Geometry check sheet. Reference: drawing and pictorial views, mm from the part's lowest x, y, z. Give positions to 0.01 mm unless a question says otherwise; leave off trailing zeros. Loops run counter-clockwise (first coordinate to the right, second up) from the corner with the lowest first, then second, coordinate; pieces in that order, holes last. Notation, with made-up numbers: (-34.5, 77.25) - (-6.5, 77.25) arc R20 ccw to (-6.5, 86.25) - close; hole circle Ø6 at (-32, 78.25). An arc over 180 degrees is marked (long way). One line per question, with ' | ' between items. Start each with the question number.
1. Section check B-B, the plane z = 22. Enter the section's corners in (x, y) (3 decimals).
2. Thickness scan on line 1 along Y through (x, z) = (22.5, 18) (3 decimals); line 2 along Y through (x, z) = (26, 12.75) (3 decimals); line 3 along X through (y, z) = (12, 10.25). Record the ranges inside material, lowest first. Write a range as from..to.
3. Section check D-D, the plane z = 13. Enter the section's corners in (x, y) (3 decimals), then the cut area to 3 significant figures.
4. Section check C-C, the plane y = 20.5. Enter the section's corners in (x, z) (3 decimals), then the cut area to 3 significant figures.
5. Mould release check, pull along Y, two halves, no side actions. Record for the marked faces 1, 2, 3 and 4: +Y half, -Y half, draft (parallel to the pull), parting line (faces both ways), or undercut.
6. Section check A-A, the plane x = 21.5. Enter the section's corners in (y, z) (3 decimals).
7. Depth check by flat-ended pin: pin 1 Ø6 at (y, z) = (16, 5.5) entering from +X. Enter the tip coordinate at first touch or a pass-through.
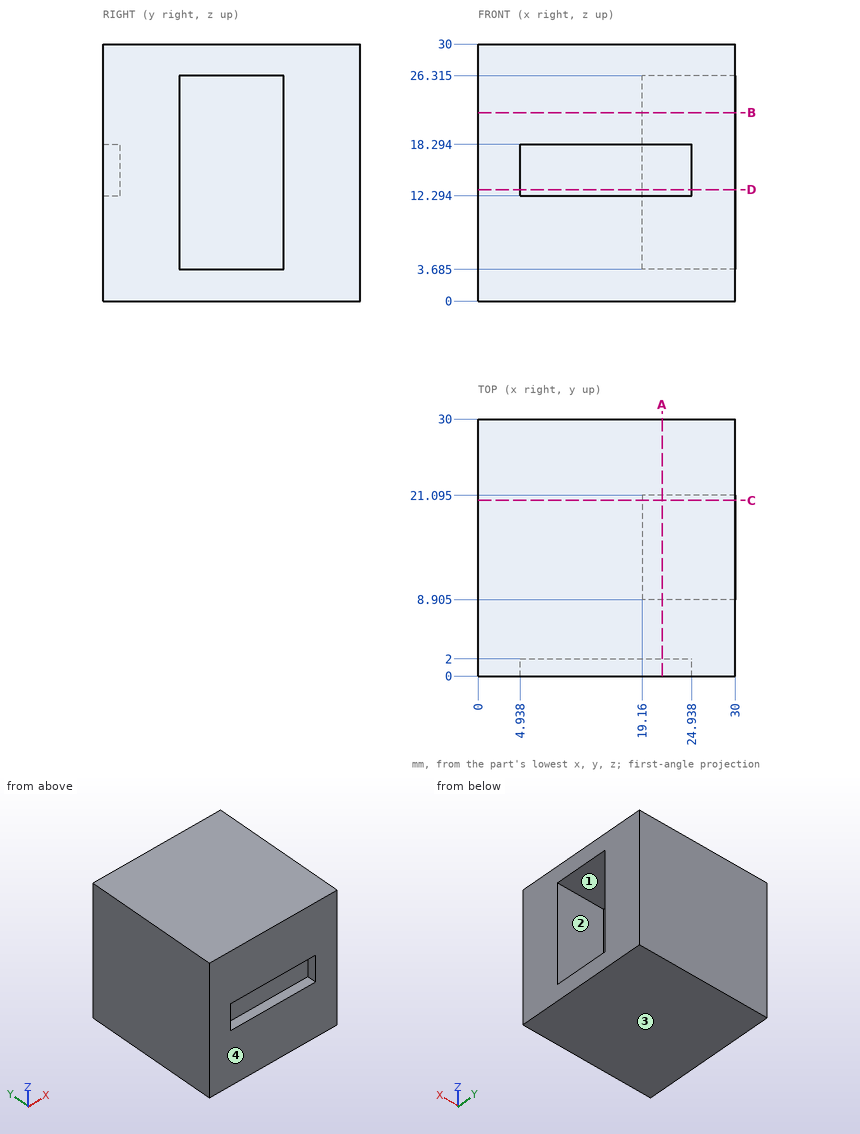
Results list:
1) outline: (0, 0) - (30, 0) - (30, 8.905) - (19.16, 8.905) - (19.16, 21.095) - (30, 21.095) - (30, 30) - (0, 30) - close
2) line 1: 2..8.905, 21.095..30 | line 2: 0..8.905, 21.095..30 | line 3: 0..19.16
3) outline: (0, 0) - (4.938, 0) - (4.938, 2) - (24.938, 2) - (24.938, 0) - (30, 0) - (30, 8.905) - (19.16, 8.905) - (19.16, 21.095) - (30, 21.095) - (30, 30) - (0, 30) - close | area: 728 mm²
4) outline: (0, 0) - (30, 0) - (30, 3.685) - (19.16, 3.685) - (19.16, 26.315) - (30, 26.315) - (30, 30) - (0, 30) - close | area: 655 mm²
5) face 1: undercut | face 2: undercut | face 3: draft | face 4: -Y half
6) outline: (0, 0) - (30, 0) - (30, 30) - (0, 30) - (0, 18.294) - (2, 18.294) - (2, 12.294) - (0, 12.294) - close; hole (8.905, 3.685) - (21.095, 3.685) - (21.095, 26.315) - (8.905, 26.315) - close
7) pin 1: x = 30
